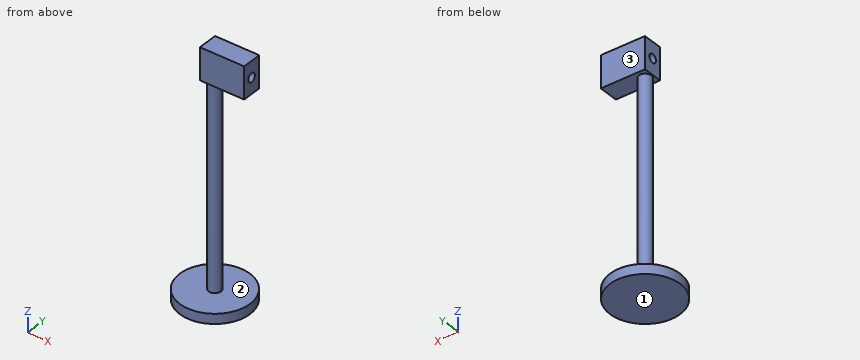
```python
from build123d import *

# Parameters (mm, degrees)
F0_R     = 28.448
F1_DEPTH = 8.001
F2_R     = 4.99999
F3_DEPTH = 165.00094
F5_DEPTH = 7.99973
F6_R     = 3.50012
F7_DEPTH = 43.9928


with BuildPart() as f1:
    # F0 (on Top) → F1 (new body)
    with BuildSketch(Plane.XY):
        Circle(F0_R)
    extrude(amount=F1_DEPTH)

    # F2 (on face) → F3 (join)
    with BuildSketch(Plane.XY.offset(8.001)):
        Circle(F2_R)
    extrude(amount=F3_DEPTH)

    # F4 (on Front) → F5 (join, symmetric)
    with BuildSketch(Plane.XZ):
        Polygon((-6.00583, 173.00194), (-4.99999, 173.00194), (4.99999, 173.00194), (29.90215, 173.00194), (29.90215, 199.00138), (-6.00583, 199.00138), align=None)
    extrude(amount=F5_DEPTH, both=True)

    # F6 (on face) → F7 (cut)
    with BuildSketch(Plane(origin=(-6.00583, 0, 0), x_dir=(0, -1, 0), z_dir=(-1, 0, 0))):
        with Locations((0.09779, 185.9026)):
            Circle(F6_R)
    extrude(amount=-F7_DEPTH, mode=Mode.SUBTRACT)


solid = f1.part
```
Verification items for the finished model (mm, model axes). Face numbers are marked on the shaded views. Coordinates: 2 decimals unless noted, no trailing zeros. Order: outer loops, then holes, each group sorted by start corner. A loop starts at its lowest first (then second) coordinate and runs counter-clockwise, first axis right, second up. Notation, with made-up numbers: (-26, 70) -> (16, 70) arc R23 cw to (16, 89) -> close; hole circle Ø11 at (85, -27). An arc over 180 degrees is marked (long way). Put each result on its own line as item: value. Start each with the question number.
1) Cross-section at B-B (y = 0). Enter the section's corners in (x, z).
2) Cross-section at A-A (x = 20.5). Enter the section's corners in (y, z), plus the area to 3 significant figures.
3) Release check for a two-part mould opening along Z. For the marked faces 1, 2 and 3 record: pulls with the +Z half, pulls with the -Z half, needs draft (parallel to the pull), parting line crosses it, or undercut.
4) Material ranges on L1, parallel to Z at x = 1, y = -5; L2, parallel to Z at x = 15, y = -1; L3, parallel to Z at x = -6, y = -17.5, recorded low to high.
5) Cross-section at D-D (z = 46.5). Enter the section's corners in (x, y), plus the area to 3 significant figures.
6) Go/stop test with flat-tipped pins: pin 1 (12 mm diameter, centred on x = -16.5, z = 135, fed in from +Y); pin 2 (21 mm diameter, centred on x = 14.5, z = 191, fed in from +Y); pin 3 (10 mm diameter, centred on x = 15.5, y = -19.5, fed in from +Z); pin 4 (4 mm diameter, centred on x = 4.5, z = 102, fed in from -Y). Record where each tip stops, or that it passes through.
7) Cross-section at C-C (x = 0). Enter the section's corners in (y, z), plus the area to 3 significant figures.
Geometry check:
1. outline: (-28.45, 0) -> (28.45, 0) -> (28.45, 8) -> (5, 8) -> (5, 173) -> (29.9, 173) -> (29.9, 182.4) -> (-6.01, 182.4) -> (-6.01, 173) -> (-5, 173) -> (-5, 8) -> (-28.45, 8) -> close; (-6.01, 189.4) -> (29.9, 189.4) -> (29.9, 199) -> (-6.01, 199) -> close
2. outline: (-19.72, 0) -> (19.72, 0) -> (19.72, 8) -> (-19.72, 8) -> close; (-8, 173) -> (8, 173) -> (8, 199) -> (-8, 199) -> close; hole circle Ø7 at (-0.1, 185.9)
2. area: 693 mm^2
3. face 1: pulls with the -Z half
3. face 2: undercut
3. face 3: needs draft
4. L1: z = 0 to 8, 173 to 199
4. L2: z = 0 to 8, 173 to 182.52, 189.28 to 199
4. L3: z = 0 to 8
5. outline: circle Ø10 at (0, 0)
5. area: 78.5 mm^2
6. pin 1: passes through
6. pin 2: stops at y = 8
6. pin 3: stops at z = 8
6. pin 4: stops at y = -4.33
7. outline: (-28.45, 0) -> (28.45, 0) -> (28.45, 8) -> (5, 8) -> (5, 173) -> (8, 173) -> (8, 199) -> (-8, 199) -> (-8, 173) -> (-5, 173) -> (-5, 8) -> (-28.45, 8) -> close; hole circle Ø7 at (-0.1, 185.9)
7. area: 2,480 mm^2
